Geometry: final body of the model. Coordinates: model frame, mm. Give positions to 0.01 mm unless a question says otherwise; leave off trailing zeros. Order: outer loops, then holes, each group sorted by start corner. A loop starts at its lowest first (then second) coordinate and runs counter-clockwise, first axis right, second up. Notation, with made-up numbers: (37, 36) - (96, 36) arc R26 cw to (96, 61) - close; hole circle Ø9 at (21.5, 62). An arc over 180 degrees is marked (long way). Put each result on its own line as item: value. Start each with the question number.
1. First-contact query: P1, Ø3, axis at y = -19, z = 6.5, coming from the -X side. Flat tip, straight axial feed; report the tip coordinate or a pass-through.
2. Section B-B on z = 0. Return the cut outline in (x, y), plus the area to 3 significant figures.
3. Mould query, pull axis Z, two halves, no side actions, for faces 1 (the flat face through (508, -13, 0)), 2 (the flat face through (250, -13, -12.7)), 3 (the flat face through (258, -13, 12.7)), 4 (the cylindrical face through (-1.55, -12.52, -6.98)). Classes: pulls with the +Z half, pulls with the -Z half, needs draft (parallel to the pull), parting line crosses it, or undercut.
4. Ray query, line 1 along X through (y, z) = (-16, -1.25); line 2 along X through (y, z) = (-9.5, 7.5); line 3 along X through (y, z) = (-8, 9.75). Return the intervals inside material, ascending. Write a range as from..to.
5. Section A-A on y = -17.25. Return the cut outline in (x, z).
from build123d import *

# Parameters (mm, degrees)
F0_R     = 7.1501
F1_DEPTH = 25.4


with BuildPart() as f1:
    # F0 (on Front) → F1 (new body)
    with BuildSketch(Plane.XZ):
        with BuildLine():
            ThreePointArc((0, 12.7), (8.980256, 8.980256), (12.7, 0))
            ThreePointArc((12.7, 0), (8.980256, -8.980256), (0, -12.7))
            Line((0, -12.7), (508, -12.7))
            Line((508, -12.7), (508, 12.7))
            Line((508, 12.7), (0, 12.7))
        make_face()
        with BuildLine():
            ThreePointArc((0, -12.7), (8.980256, -8.980256), (12.7, 0))
            ThreePointArc((12.7, 0), (8.980256, 8.980256), (0, 12.7))
            ThreePointArc((0, 12.7), (-12.7, 0), (0, -12.7))
        make_face()
        Circle(F0_R, mode=Mode.SUBTRACT)
    extrude(amount=F1_DEPTH)


solid = f1.part
Resolved:
1. P1: x = -11.67
2. outline: (-12.7, -25.4) - (-7.15, -25.4) - (-7.15, 0) - (-12.7, 0) - close; (7.15, -25.4) - (508, -25.4) - (508, 0) - (7.15, 0) - close
2. area: 12,900 mm^2
3. face 1: needs draft
3. face 2: pulls with the -Z half
3. face 3: pulls with the +Z half
3. face 4: undercut
4. line 1: -12.64..-7.04, 7.04..508
4. line 2: -10.25..508
4. line 3: -8.14..508
5. outline: (0, -12.7) - (508, -12.7) - (508, 12.7) - (0, 12.7) arc R12.7 ccw to start; hole circle Ø14.3 at (0, 0)
